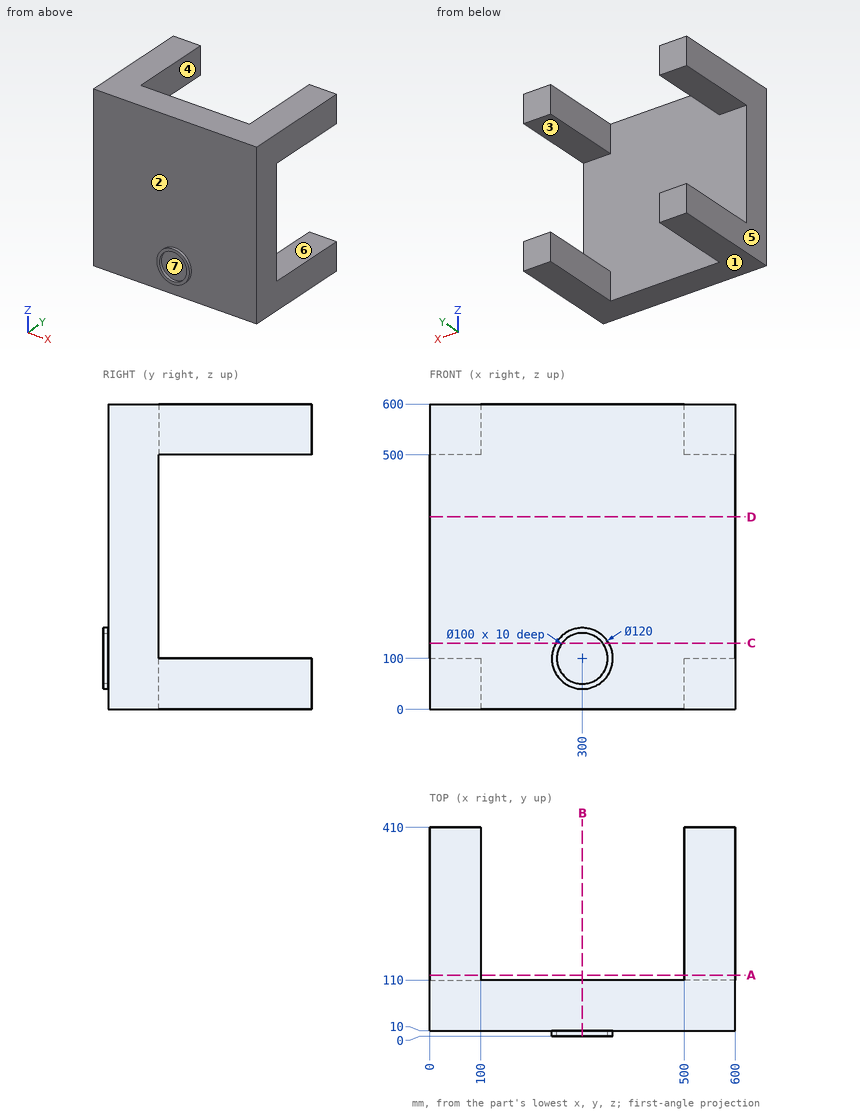
Print and shaded views of the part. All mm, measured from the part's lowest x, y and z. A direction names the side the tool comes from. Coordinates: 2 decimals unless noted, no trailing zeros. Order: outer loops, then holes, each group sorted by start corner. A loop starts at its lowest first (then second) coordinate and runs counter-clockwise, first axis right, second up. Notation, with made-up numbers: (26, 5.25) -> (56, 5.25) arc R30 cw to (56, 40.25) -> close; hole circle Ø8 at (78, -8.5). An arc over 180 degrees is marked (long way). Answer as a JSON object with one key per item and string values. Group by question number.
1) Cut at B-B, the plane x = 300. Write the cut outline in (y, z).
2) Cut at A-A, the plane y = 119.5. Write the cut outline in (x, z), then the cut area to 3 significant figures.
3) Cut at D-D, the plane z = 378. Write the cut outline in (x, y), then the cut area to 3 significant figures.
4) Drill centre lines: L1, parallel to X at y = 247, z = 547; L2, parallel to X at y = 7, z = 100. Where is each one in solid material? Low to high.
5) Cut at C-C, the plane z = 130. Write the cut outline in (x, y).
6) Which spindle directions (+Z, -Z, +X, -X, +Y, -Y) get a long thin tool onto all of the face, cutting with end or side? Do the marked faces 4, 5, 6 and 7. Say none if no direction does.
7) Pull direction Z, two halves, no side cores. Call the marked faces 1, 2 and 3: +Z half, -Z half, draft (parallel to the pull), parting line (faces both ways), or undercut.
8) Flat gauge pin, fed straight in: pin 1 (4 mm diameter, centred on x = 472, z = 232, fed in from +Y). Where does the tip first touch, or does it go through?
Check values:
{
 "1": {"outline": "(0, 40) -> (10, 40) -> (10, 0) -> (110, 0) -> (110, 600) -> (10, 600) -> (10, 160) -> (0, 160) -> (0, 150) -> (10, 150) -> (10, 50) -> (0, 50) -> close"},
 "2": {"outline": "(0, 0) -> (100, 0) -> (100, 100) -> (0, 100) -> close; (0, 500) -> (100, 500) -> (100, 600) -> (0, 600) -> close; (500, 0) -> (600, 0) -> (600, 100) -> (500, 100) -> close; (500, 500) -> (600, 500) -> (600, 600) -> (500, 600) -> close", "area": "40,000 mm²"},
 "3": {"outline": "(0, 10) -> (600, 10) -> (600, 110) -> (0, 110) -> close", "area": "60,000 mm²"},
 "4": {"L1": "x = 0 to 100, 500 to 600", "L2": "x = 240 to 250, 350 to 360"},
 "5": {"outline": "(0, 10) -> (248.04, 10) -> (248.04, 0) -> (260, 0) -> (260, 10) -> (340, 10) -> (340, 0) -> (351.96, 0) -> (351.96, 10) -> (600, 10) -> (600, 110) -> (0, 110) -> close"},
 "6": {"face 4": "+Z, -Z, +Y", "face 5": "+Z, -Z, -X, +Y, -Y", "face 6": "+X, -X, +Y", "face 7": "-Y"},
 "7": {"face 1": "-Z half", "face 2": "draft", "face 3": "undercut"},
 "8": {"pin 1": "stops at y = 110"}
}
